Work out the finished part from the listing and answer in its coordinate system (mm). A direction names the side the tool comes from. Coordinates: 2 decimals unless noted, no trailing zeros. Write each loop counter-clockwise with the first axis right and the second up, starting at its lowest first coordinate (ties: lowest second). Pieces come first, ordered by that corner, then holes. Notation, with made-up numbers: M 68,4.5 L 126,4.5 A12 cw 126,21.5 Z; hole C 58.5,53 d11. An arc over 180 degrees is marked long. Use CSV: the item, a comma, the result in double quotes.
from build123d import *

# Parameters (mm, degrees)
BOSS_EXTRUDE1_DEPTH = 10
BOSS_EXTRUDE2_DEPTH = 100
SKETCH4_R           = 5
CUT_EXTRUDE1_DEPTH  = 10


with BuildPart() as part:
    # Sketch2 → Boss-Extrude1 (new body)
    with BuildSketch(Plane(origin=(0, 0, 0), x_dir=(1, 0, 0), z_dir=(0, 1, 0))):
        Polygon((-60, -80), (-60, -20), (60, -20), (60, -80), (100, -80), (100, 80), (-100, 80), (-100, -80), align=None)
    extrude(amount=BOSS_EXTRUDE1_DEPTH)

    # Sketch3 → Boss-Extrude2 (add)
    with BuildSketch(Plane(origin=(0, 10, 0), x_dir=(1, 0, 0), z_dir=(0, 1, 0))):
        Polygon((-60, -80), (-60, -20), (60, -20), (60, -80), (100, -80), (100, 80), (-100, 80), (-100, -80), align=None)
        Polygon((90, 70), (-90, 70), (-90, -70), (-70, -70), (-70, -10), (70, -10), (70, -70), (90, -70), align=None, mode=Mode.SUBTRACT)
    extrude(amount=BOSS_EXTRUDE2_DEPTH)

    # Sketch4 → Cut-Extrude1 (cut)
    with BuildSketch(Plane(origin=(0, 10, 0), x_dir=(1, 0, 0), z_dir=(0, 1, 0))):
        with Locations((0, 23.078006165)):
            Circle(SKETCH4_R)
    extrude(amount=-CUT_EXTRUDE1_DEPTH, mode=Mode.SUBTRACT)


solid = part.part
Item 1: The part is cut by section A-A (y = 72.5). Write down the section's boundary in (x, z), then the cut area to 3 significant figures.
Answer:
outline,"M -100,-80 L 100,-80 L 100,80 L 60,80 L 60,20 L -60,20 L -60,80 L -100,80 Z; hole M -90,-70 L 90,-70 L 90,70 L 70,70 L 70,10 L -70,10 L -70,70 L -90,70 Z"
area,"8,000 mm2"
Item 2: The part is cut by section C-C (x = 0). Write down the section's boundary in (y, z).
Answer:
outline,"M 0,-80 L 110,-80 L 110,-70 L 10,-70 L 10,-28.08 L 0,-28.08 Z; M 0,-18.08 L 10,-18.08 L 10,10 L 110,10 L 110,20 L 0,20 Z"
Item 3: For a pull along Z with two mould halves and no side action, classify faces 4 (the face through (80, 59, 70)), 5 (the face through (-60, 54, 50)), 6 (the face through (80, 54, 80)) as released by +Z, released by -Z, zero draft, split by the parting line, or undercut.
Answer:
face 4,"undercut"
face 5,"zero draft"
face 6,"released by +Z"
Item 4: Given pin 1 (5 mm diameter, centred on x = 7.5, z = 24, fed in from +Y); pin 2 (11.5 mm diameter, centred on x = 0, z = -23.08, fed in from +Y), each flat-ended and moving along its own axis, determine where each tip first touches the part or whether it passes through.
Answer:
pin 1,"passes through"
pin 2,"stops at y = 10"
Item 5: The part is cut by section D-D (z = -64). Write down the section's boundary in (x, y), then the cut area to 3 significant figures.
Answer:
outline,"M -100,0 L 100,0 L 100,110 L 90,110 L 90,10 L -90,10 L -90,110 L -100,110 Z"
area,"4,000 mm2"
Item 6: A tool of negligible diameter and unlimited length cuts with its end or side. For faces 1 (the face through (-1, 0, -1)), 2 (the face through (-80, 59, 70)), 3 (the face through (-1, 54, 20)), from which of +Z, -Z, +X, -X, +Y, -Y can it reach the whole face along a straight path? Write none if from no direction.
Answer:
face 1,"+Z, -Z, +X, -X, -Y"
face 2,"+Y"
face 3,"+Z, +Y, -Y"
Item 7: The part is cut by section B-B (z = 42.5). Write down the section's boundary in (x, y).
Answer:
outline,"M -100,0 L -60,0 L -60,110 L -70,110 L -70,10 L -90,10 L -90,110 L -100,110 Z; M 60,0 L 100,0 L 100,110 L 90,110 L 90,10 L 70,10 L 70,110 L 60,110 Z"
Item 8: Consider probe 1 along X at (y, z) = (43.5, 68); probe 2 along X at (y, z) = (76, 18.5); probe 3 along X at (y, z) = (31, -15.5). Determine where each line is inside the solid, lowest interval first.
Answer:
probe 1,"x = -100 to -90, -70 to -60, 60 to 70, 90 to 100"
probe 2,"x = -100 to -90, -70 to 70, 90 to 100"
probe 3,"x = -100 to -90, 90 to 100"
